from build123d import *

# Parameters (mm, degrees)
BOSS_EXTRUDE1_DEPTH     = 31.75
BOSS_EXTRUDE2_DEPTH     = 6.35
CUT_EXTRUDE2_DEPTH      = 6.4135
BOSS_EXTRUDE3_START     = 28.702
BOSS_EXTRUDE3_DEPTH     = 3.048
BOSS_EXTRUDE5_START     = -31.75
BOSS_EXTRUDE5_DEPTH     = 3.048
BOSS_EXTRUDE7_START     = 21.717
BOSS_EXTRUDE7_DEPTH     = 3.175
BOSS_EXTRUDE8_START     = -21.717
BOSS_EXTRUDE8_DEPTH     = 3.175
BOSS_EXTRUDE6_START     = 31.75
BOSS_EXTRUDE6_DEPTH     = 13.208
BOSS_EXTRUDE9_START     = -31.75
BOSS_EXTRUDE9_DEPTH     = 13.208
SKETCH3_W               = 15.24
SKETCH3_H               = 15.875
CUT_EXTRUDE4_DEPTH      = 11.31875
CUT_EXTRUDE4_DEPTH_BACK = 3.38125
SKETCH5_W               = 50.8
SKETCH5_H               = 1.74625
CUT_EXTRUDE6_DEPTH      = 6.35
SKETCH6_W               = 9.525
SKETCH6_H               = 1.905
CUT_EXTRUDE7_DEPTH      = 1.905


with BuildPart() as part:
    # Sketch1 → Boss-Extrude1 (new body, symmetric)
    with BuildSketch(Plane.XY):
        Polygon((-25.4, -0.79375), (-25.4, 3.175), (-28.575, 3.175), (-28.575, -3.175), (28.575, -3.175), (28.575, 3.175), (25.4, 3.175), (25.4, -0.79375), align=None)
    extrude(amount=BOSS_EXTRUDE1_DEPTH, both=True)

    # Sketch1<3> → Boss-Extrude2 (add, symmetric)
    with BuildSketch(Plane.XY):
        with BuildLine():
            Line((23.8125, 9.525), (23.8125, -0.79375))
            Line((23.8125, -0.79375), (25.4, -0.79375))
            Line((25.4, -0.79375), (25.4, 5.588))
            Line((25.4, 5.588), (26.543, 5.588))
            ThreePointArc((26.543, 5.588), (26.761343, 5.712222), (26.766119, 5.963383))
            Line((26.766119, 5.963383), (24.8285, 9.525))
            Line((24.8285, 9.525), (23.8125, 9.525))
        make_face()
    extrude(amount=BOSS_EXTRUDE2_DEPTH, both=True)

    # Sketch1<6> → Cut-Extrude2 (cut, symmetric)
    with BuildSketch(Plane.XY):
        with BuildLine():
            Line((26.035, 3.175), (25.4, 3.175))
            Line((25.4, 3.175), (25.4, -0.79375))
            Line((25.4, -0.79375), (25.4, -2.06375))
            ThreePointArc((25.4, -2.06375), (25.7175, -2.38125), (26.035, -2.06375))
            Line((26.035, -2.06375), (26.035, 3.175))
        make_face()
    extrude(amount=CUT_EXTRUDE2_DEPTH, both=True, mode=Mode.SUBTRACT)

    # Cut-Sweep1: sweep along a path in Sketch7
    with BuildLine(Plane(origin=(0, -0.79375, 0), x_dir=(1, 0, 0), z_dir=(0, 1, 0))) as cut_sweep1_path:
        Line((26.035, 6.35), (23.9395, 6.35))
        ThreePointArc((23.9395, 6.35), (23.849697, 6.312803), (23.8125, 6.223))
        Line((23.8125, 6.223), (23.8125, -6.223))
        ThreePointArc((23.8125, -6.223), (23.849697, -6.312803), (23.9395, -6.35))
        Line((23.9395, -6.35), (26.035, -6.35))
    # Sketch8 → Cut-Sweep1 (sweep, cut)
    with BuildSketch(Plane(origin=(26.035, 0, 0), x_dir=(0, 0, -1), z_dir=(1, 0, 0))):
        with BuildLine():
            Line((-6.858, -2.69875), (-6.858, 9.525))
            Line((-6.858, 9.525), (-6.35, 9.525))
            Line((-6.35, 9.525), (-6.35, -2.69875))
            ThreePointArc((-6.35, -2.69875), (-6.604, -2.95275), (-6.858, -2.69875))
        make_face()
    sweep(path=cut_sweep1_path.line, mode=Mode.SUBTRACT)

    # Sketch1<7> → Boss-Extrude3 (add)
    with BuildSketch(Plane.XY.offset(BOSS_EXTRUDE3_START)):
        with BuildLine():
            ThreePointArc((-32.355812, 1.550246), (-32.476313, 2.608154), (-31.574994, 3.175))
            Line((-31.574994, 3.175), (-28.575, 3.175))
            Line((-28.575, 3.175), (-28.575, -3.175))
            Line((-28.575, -3.175), (-32.355812, 1.550246))
        make_face()
        with BuildLine():
            ThreePointArc((-30.574996, 2.175002), (-30.867889, 2.882107), (-31.574994, 3.175))
            ThreePointArc((-31.574994, 3.175), (-32.476313, 2.608154), (-32.355812, 1.550246))
            ThreePointArc((-32.355812, 1.550246), (-31.24395, 1.231389), (-30.574996, 2.175002))
        make_face()
    extrude(amount=BOSS_EXTRUDE3_DEPTH)

    # Sketch1<9> → Boss-Extrude5 (add)
    with BuildSketch(Plane.XY.offset(BOSS_EXTRUDE5_START)):
        with BuildLine():
            ThreePointArc((-32.355812, 1.550246), (-32.476313, 2.608154), (-31.574994, 3.175))
            Line((-31.574994, 3.175), (-28.575, 3.175))
            Line((-28.575, 3.175), (-28.575, -3.175))
            Line((-28.575, -3.175), (-32.355812, 1.550246))
        make_face()
        with BuildLine():
            ThreePointArc((-30.574996, 2.175002), (-30.867889, 2.882107), (-31.574994, 3.175))
            ThreePointArc((-31.574994, 3.175), (-32.476313, 2.608154), (-32.355812, 1.550246))
            ThreePointArc((-32.355812, 1.550246), (-31.24395, 1.231389), (-30.574996, 2.175002))
        make_face()
    extrude(amount=BOSS_EXTRUDE5_DEPTH)

    # Sketch1<13> → Boss-Extrude7 (add)
    with BuildSketch(Plane.XY.offset(BOSS_EXTRUDE7_START)):
        with BuildLine():
            Line((-28.575, -3.175), (-28.575, 3.175))
            Line((-28.575, 3.175), (-31.574994, 3.175))
            ThreePointArc((-31.574994, 3.175), (-30.867889, 2.882107), (-30.574996, 2.175002))
            ThreePointArc((-30.574996, 2.175002), (-31.24395, 1.231389), (-32.355812, 1.550246))
            Line((-32.355812, 1.550246), (-28.575, -3.175))
        make_face()
        with BuildLine():
            ThreePointArc((-30.574996, 2.175002), (-30.867889, 2.882107), (-31.574994, 3.175))
            ThreePointArc((-31.574994, 3.175), (-32.476313, 2.608154), (-32.355812, 1.550246))
            ThreePointArc((-32.355812, 1.550246), (-31.24395, 1.231389), (-30.574996, 2.175002))
        make_face()
    extrude(amount=-BOSS_EXTRUDE7_DEPTH)

    # Sketch1<14> → Boss-Extrude8 (add)
    with BuildSketch(Plane.XY.offset(BOSS_EXTRUDE8_START)):
        with BuildLine():
            Line((-28.575, -3.175), (-28.575, 3.175))
            Line((-28.575, 3.175), (-31.574994, 3.175))
            ThreePointArc((-31.574994, 3.175), (-30.867889, 2.882107), (-30.574996, 2.175002))
            ThreePointArc((-30.574996, 2.175002), (-31.24395, 1.231389), (-32.355812, 1.550246))
            Line((-32.355812, 1.550246), (-28.575, -3.175))
        make_face()
        with BuildLine():
            ThreePointArc((-30.574996, 2.175002), (-30.867889, 2.882107), (-31.574994, 3.175))
            ThreePointArc((-31.574994, 3.175), (-32.476313, 2.608154), (-32.355812, 1.550246))
            ThreePointArc((-32.355812, 1.550246), (-31.24395, 1.231389), (-30.574996, 2.175002))
        make_face()
    extrude(amount=BOSS_EXTRUDE8_DEPTH)

    # Sketch1<10> → Boss-Extrude6 (add)
    with BuildSketch(Plane.XY.offset(BOSS_EXTRUDE6_START)):
        with BuildLine():
            ThreePointArc((-30.574996, 2.175002), (-30.867889, 2.882107), (-31.574994, 3.175))
            ThreePointArc((-31.574994, 3.175), (-32.476313, 2.608154), (-32.355812, 1.550246))
            ThreePointArc((-32.355812, 1.550246), (-31.24395, 1.231389), (-30.574996, 2.175002))
        make_face()
    extrude(amount=-BOSS_EXTRUDE6_DEPTH)

    # Sketch1<16> → Boss-Extrude9 (add)
    with BuildSketch(Plane.XY.offset(BOSS_EXTRUDE9_START)):
        with BuildLine():
            ThreePointArc((-30.574996, 2.175002), (-30.867889, 2.882107), (-31.574994, 3.175))
            ThreePointArc((-31.574994, 3.175), (-32.476313, 2.608154), (-32.355812, 1.550246))
            ThreePointArc((-32.355812, 1.550246), (-31.24395, 1.231389), (-30.574996, 2.175002))
        make_face()
    extrude(amount=BOSS_EXTRUDE9_DEPTH)

    # Sketch3 → Cut-Extrude4 (cut, two sides)
    with BuildSketch(Plane(origin=(0, -0.79375, 0), x_dir=(1, 0, 0), z_dir=(0, 1, 0))) as cut_extrude4_sk:
        with Locations((10.795, 11.1125)):
            Rectangle(SKETCH3_W, SKETCH3_H)
        with Locations((-10.795, 11.1125)):
            Rectangle(SKETCH3_W, SKETCH3_H)
        with Locations((10.795, -11.1125)):
            Rectangle(SKETCH3_W, SKETCH3_H)
        with Locations((-10.795, -11.1125)):
            Rectangle(SKETCH3_W, SKETCH3_H)
    extrude(amount=CUT_EXTRUDE4_DEPTH, mode=Mode.SUBTRACT)
    extrude(cut_extrude4_sk.sketch, amount=-CUT_EXTRUDE4_DEPTH_BACK, mode=Mode.SUBTRACT)

    # Sketch5 → Cut-Extrude6 (cut)
    with BuildSketch(Plane.XY.offset(31.75)):
        with Locations((0, -1.666875)):
            Rectangle(SKETCH5_W, SKETCH5_H)
    cut_extrude6 = extrude(amount=-CUT_EXTRUDE6_DEPTH, mode=Mode.SUBTRACT)

    # Mirror1: Cut-Extrude6 across plane
    add(cut_extrude6.mirror(Plane.XY), mode=Mode.SUBTRACT)

    # Sketch6 → Cut-Extrude7 (cut)
    with BuildSketch(Plane(origin=(28.575, 0, 0), x_dir=(0, 0, -1), z_dir=(1, 0, 0))):
        with Locations((-23.8125, 2.2225)):
            Rectangle(SKETCH6_W, SKETCH6_H)
        with Locations((23.8125, 2.2225)):
            Rectangle(SKETCH6_W, SKETCH6_H)
    extrude(amount=-CUT_EXTRUDE7_DEPTH, mode=Mode.SUBTRACT)


solid = part.part
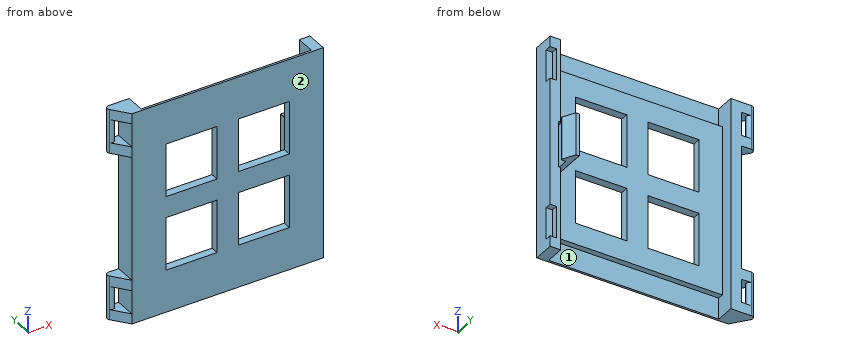
Read the model definition and answer for the solid it produces. Units are mm, in the model's axes. Face numbers are marked on the shaded views. Round coordinates to 2 decimals unless told otherwise and drop trailing zeros. Loops run counter-clockwise (first coordinate to the right, second up) from the corner with the lowest first, then second, coordinate; pieces in that order, holes last. Notation, with made-up numbers: (-14, 63.25) - (44, 63.25) arc R17 cw to (44, 94.25) - close; hole circle Ø1 at (-9.75, 83). An arc over 180 degrees is marked (long way). One line per question, with ' | ' between items. Start each with the question number.
Q1. Section A-A on x = -5.5 is taken. Give the vertices of the cut face in (y, z) (3 decimals), plus the area to 3 significant figures.
Q2. Section D-D on y = 6.75 is taken. Give the vertices of the cut face in (x, z).
Q3. Flat-ended cylindrical pins translate along their axes: pin 1 (5 mm diameter, centred on x = 2.5, z = -8.5, fed in from +Y); pin 2 (1.5 mm diameter, centred on y = 5, z = -20.5, fed in from -X); pin 3 (1.9 mm diameter, centred on x = 12, y = -1.5, fed in from +Z); pin 4 (1.9 mm diameter, centred on y = -1.5, z = -8, fed in from -X) (3 decimals). Find the tip coordinate at first contact, or state that the pin passes through.
Q4. Find the intervals of material crossed by L1, parallel to Z at x = -7.5, y = -2 (3 decimals); L2, parallel to Z at x = 25.5, y = -2.5; L3, parallel to X at y = -0.75, z = 10.5 (3 decimals), in increasing order.
Q5. Section B-B on z = 13.5 is taken. Give the vertices of the cut face in (x, y) (3 decimals).
Q6. Section C-C on x = -22 is taken. Give the vertices of the cut face in (y, z) (3 decimals).
Q7. For a pull along X with two mould halves and no side action, classify the marked faces 1 and 2 as +X half, -X half, draft (parallel to the pull), parting line (faces both ways), or undercut.
Established:
1) outline: (-3.175, -31.75) - (-2.54, -31.75) - (-2.54, -25.4) - (-0.794, -25.4) - (-0.794, -19.05) - (-3.175, -19.05) - close; (-3.175, -3.175) - (-0.794, -3.175) - (-0.794, 3.175) - (-3.175, 3.175) - close; (-3.175, 19.05) - (-0.794, 19.05) - (-0.794, 25.4) - (-2.54, 25.4) - (-2.54, 31.75) - (-3.175, 31.75) - close | area: 53.4 mm²
2) outline: (23.81, -6.22) arc R0.13 ccw to (23.94, -6.35) - (26.34, -6.35) - (26.34, 6.35) - (23.94, 6.35) arc R0.13 ccw to (23.81, 6.22) - close
3) pin 1: y = -0.79 | pin 2: through | pin 3: z = 25.4 | pin 4: x = -28.575
4) L1: -25.4 to -19.05, -3.175 to 3.175, 19.05 to 25.4 | L2: -31.75 to -6.86, -6.35 to 6.35, 6.86 to 31.75 | L3: -28.575 to -25.4, 25.4 to 28.575
5) outline: (-28.575, -3.175) - (-18.415, -3.175) - (-18.415, -0.794) - (-25.4, -0.794) - (-25.4, 3.175) - (-28.575, 3.175) - close; (-3.175, -3.175) - (3.175, -3.175) - (3.175, -0.794) - (-3.175, -0.794) - close; (18.415, -3.175) - (28.575, -3.175) - (28.575, 3.175) - (25.4, 3.175) - (25.4, -0.794) - (18.415, -0.794) - close
6) outline: (-3.175, -31.75) - (-2.54, -31.75) - (-2.54, -25.4) - (-0.794, -25.4) - (-0.794, 25.4) - (-2.54, 25.4) - (-2.54, 31.75) - (-3.175, 31.75) - close
7) face 1: undercut | face 2: draft
